from build123d import *

# Parameters (mm, degrees)
BOSS_EXTRUDE1_DEPTH = 15.24


with BuildPart() as part:
    # Sketch1 → Boss-Extrude1 (new body)
    with BuildSketch(Plane(origin=(0, 0, 0), x_dir=(0, 0, -1), z_dir=(1, 0, 0))):
        with BuildLine():
            Line((-0.6, 6.665999974), (-0.6, 7.285861192))
            Line((-0.6, 7.285861192), (-1.46058835, 7.285861192))
            Line((-1.46058835, 7.285861192), (-4.476578637, -1.101757214))
            ThreePointArc((-4.476578637, -1.101757214), (-4.402791775, -1.649877187), (-3.911970022, -1.904777192))
            Line((-3.911970022, -1.904777192), (3.911970022, -1.904777192))
            ThreePointArc((3.911970022, -1.904777192), (4.402791775, -1.649877187), (4.476578637, -1.101757214))
            Line((4.476578637, -1.101757214), (1.46058835, 7.285861192))
            Line((1.46058835, 7.285861192), (0.6, 7.285861192))
            Line((0.6, 7.285861192), (0.6, 6.665999974))
            ThreePointArc((0.6, 6.665999974), (1, 6.265999974), (0.6, 5.865999974))
            Line((0.6, 5.865999974), (0.6, 5.246138756))
            Line((0.6, 5.246138756), (2.197641003, 0.803019978))
            ThreePointArc((2.197641003, 0.803019978), (2.12385414, 0.254900005), (1.633032387, 0))
            Line((1.633032387, 0), (0, 0))
            Line((0, 0), (-1.633032387, 0))
            ThreePointArc((-1.633032387, 0), (-2.12385414, 0.254900005), (-2.197641003, 0.803019978))
            Line((-2.197641003, 0.803019978), (-0.6, 5.246138756))
            Line((-0.6, 5.246138756), (-0.6, 5.865999974))
            ThreePointArc((-0.6, 5.865999974), (-1, 6.265999974), (-0.6, 6.665999974))
        make_face()
    extrude(amount=BOSS_EXTRUDE1_DEPTH)


solid = part.part
The model under review builds one solid part; all positions refer to its coordinate system, in mm. A direction names the side the tool comes from. Give positions to 0.01 mm unless a question says otherwise; leave off trailing zeros. Write each loop counter-clockwise with the first axis right and the second up, starting at its lowest first coordinate (ties: lowest second). Pieces come first, ordered by that corner, then holes. Notation, with made-up numbers: M -38,-26 L 3,-26 A8 cw 3,-13 Z; hole C 11,-15 d8. An arc over 180 degrees is marked long. One line per question, with ' | ' between items. Start each with the question number.
Item 1: Draft analysis for pull direction Y (two halves, no side actions). For faces 3 (the flat face through (8, 3, -3)), 4 (the flat face through (8, -1.905, 0)), 5 (the flat face through (7.51, 2.99, 1.41)), state which applies: released by +Y, released by -Y, zero draft, split by the parting line, or undercut.
Item 2: We need section D-D on z = 0.25. Write out the cut boundary in (x, y), plus the area to 3 significant figures.
Item 3: Wall thickness on line 1 (Z direction, x = 11.25, y = -1.25); line 2 (Y direction, x = 5.5, z = -0.25); line 3 (Z direction, x = 7, y = 3.5): over which ranges is each line inside the solid? List them lowest first. Write a range as from..to.
Item 4: We need section C-C on y = 0.25. Write out the cut boundary in (x, z).
Item 5: We need section B-B on x = 9.5. Write out the cut boundary in (y, z).
Item 6: For faces 1 (the flat face through (15.24, -0.3, 0.1)), 2 (the cylindrical face through (7.513, 0.262, -2.128)), list the 3-axis set-ups (+Z, -Z, +X, -X, +Y, -Y) from which the entire face can be reached by the end or side of a thin tool; tool diameter is ignored.
Item 7: We need section A-A on y = 5. Write out the cut boundary in (x, z).
Item 8: For pin 1 (0.5 mm diameter, centred on x = 11, y = 7, fed in from +Z); pin 2 (4 mm diameter, centred on x = 2.5, y = 3, fed in from +Z); pin 3 (0.7 mm diameter, centred on x = 6, y = 5.5, fed in from -Z), all flat-tipped, find the tip position at first contact; note any pin that passes through.
Results found:
1) face 3: released by +Y | face 4: released by -Y | face 5: undercut
2) outline: M 0,-1.9 L 15.24,-1.9 L 15.24,0 L 0,0 Z | area: 29.0 mm2
3) line 1: z = -4.51..4.51 | line 2: y = -1.9..0 | line 3: z = -2.82..-1.23, 1.23..2.82
4) outline: M 0,-3.99 L 15.24,-3.99 L 15.24,-2.12 L 0,-2.12 Z; M 0,2.12 L 15.24,2.12 L 15.24,3.99 L 0,3.99 Z
5) outline: M -1.9,-3.91 A0.6 ccw -1.1,-4.48 L 7.29,-1.46 L 7.29,-0.6 L 6.67,-0.6 A0.4 cw 5.87,-0.6 L 5.25,-0.6 L 0.8,-2.2 A0.6 cw 0,-1.63 L 0,1.63 A0.6 cw 0.8,2.2 L 5.25,0.6 L 5.87,0.6 A0.4 cw 6.67,0.6 L 7.29,0.6 L 7.29,1.46 L -1.1,4.48 A0.6 ccw -1.9,3.91 Z
6) face 1: +Z, -Z, +X, +Y, -Y | face 2: +X, -X
7) outline: M 0,-2.28 L 15.24,-2.28 L 15.24,-0.69 L 0,-0.69 Z; M 0,0.69 L 15.24,0.69 L 15.24,2.28 L 0,2.28 Z
8) pin 1: stops at z = 1.65 | pin 2: stops at z = 3.72 | pin 3: stops at z = -2.23
